Source: CAD feature listing. Evaluate the final solid. Frame: model axes, mm. A direction names the side the tool comes from. Round coordinates to 2 decimals unless told otherwise and drop trailing zeros. Loops run counter-clockwise (first coordinate to the right, second up) from the corner with the lowest first, then second, coordinate; pieces in that order, holes last.
Item 1: Pull-direction query (Z, two-part tool) for faces 1 (the cylindrical face through (15, -21, 28)), 2 (the flat face through (25, 5, 0)), 3 (the flat face through (0, 0, 0)); classes: released by +Z, released by -Z, zero draft, split by the parting line, or undercut.
Item 2: Ray query, L1, parallel to Y at x = 13, z = 0; L2, parallel to Y at x = 27.45, z = 0; L3, parallel to Z at x = 5, y = 5. Return the intervals inside material, ascending.
Item 3: Section query D-D on x = 19.25. Return loops of the section in (y, z), then the cut area to 3 significant figures.
Item 4: Access query for faces 4 (the flat face through (30, -7.3, -7.3)), 5 (the cylindrical face through (27.54, -9.76, 2.17)). Directions: +Z, -Z, +X, -X, +Y, -Y. A direction counts if a zero-diameter tool reaches every point of the face in a straight line with its end or side. Return the directions, or none.
Item 5: Section query B-B on z = 0. Return loops of the section in (x, y), then the cut area to 3 significant figures.
Item 6: Section query A-A on y = 0. Return loops of the section in (x, z).
Item 7: First-contact query: P1, Ø3, axis at x = 7, z = -9.5, coming from the +Y side; P2, Ø10, axis at x = 4, z = -12, coming from the -Y side; P3, Ø18, axis at y = 0, z = 0, coming from the +X side. Flat tips, straight axial feed; report the tip coordinate or a pass-through.
Item 8: Section query C-C on x = 5.5. Return loops of the section in (y, z).
```python
from build123d import *

# Parameters (mm, degrees)
SKETCH1_R           = 35
BOSS_EXTRUDE1_DEPTH = 30
SKETCH2_R           = 10
CUT_EXTRUDE1_DEPTH  = 5
CUT_EXTRUDE2_DEPTH  = 15


with BuildPart() as part:
    # Sketch1 → Boss-Extrude1 (new body)
    with BuildSketch(Plane(origin=(0, 0, 0), x_dir=(0, 0, -1), z_dir=(1, 0, 0))):
        Circle(SKETCH1_R)
    extrude(amount=BOSS_EXTRUDE1_DEPTH)

    # Sketch2 → Cut-Extrude1 (cut)
    with BuildSketch(Plane(origin=(30, 0, 0), x_dir=(0, 0, -1), z_dir=(1, 0, 0))):
        Circle(SKETCH2_R)
    extrude(amount=-CUT_EXTRUDE1_DEPTH, mode=Mode.SUBTRACT)

    # Sketch3 → Cut-Extrude2 (cut)
    with BuildSketch(Plane(origin=(25, 0, 0), x_dir=(0, 0, -1), z_dir=(1, 0, 0))):
        with BuildLine():
            Line((-6.92820323, 4), (6.92820323, 4))
            ThreePointArc((6.92820323, 4), (0, -8), (-6.92820323, 4))
        make_face()
    extrude(amount=-CUT_EXTRUDE2_DEPTH, mode=Mode.SUBTRACT)


solid = part.part
```
Data:
1. face 1: split by the parting line
1. face 2: undercut
1. face 3: zero draft
2. L1: y = -35 to -8, 4 to 35
2. L2: y = -35 to -10, 10 to 35
2. L3: z = -34.64 to 34.64
3. outline: circle Ø70 at (0, 0); hole (4, -6.93) - (4, 6.93) arc R8 ccw (long way) to start
3. area: 3,690 mm2
4. face 4: +Z, -Z, +X, +Y, -Y
4. face 5: +X
5. outline: (0, -35) - (30, -35) - (30, -10) - (25, -10) - (25, -8) - (10, -8) - (10, 4) - (25, 4) - (25, 10) - (30, 10) - (30, 35) - (0, 35) - close
5. area: 1,820 mm2
6. outline: (0, -35) - (30, -35) - (30, -10) - (25, -10) - (25, -8) - (10, -8) - (10, 8) - (25, 8) - (25, 10) - (30, 10) - (30, 35) - (0, 35) - close
7. P1: stops at y = 34.07
7. P2: stops at y = -34.29
7. P3: stops at x = 25
8. outline: circle Ø70 at (0, 0)
